```python
from build123d import *

# Parameters (mm, degrees)
BOSS_EXTRUDE1_DEPTH = 6.35
SKETCH2_W           = 17.78
SKETCH2_H           = 8.89
CUT_EXTRUDE1_DEPTH  = 6.35
SKETCH3_W           = 6.35
SKETCH3_H           = 6.35
BOSS_EXTRUDE2_DEPTH = 12.7


with BuildPart() as part:
    # Sketch1 → Boss-Extrude1 (new body)
    with BuildSketch(Plane(origin=(0, 0, 0), x_dir=(1, 0, 0), z_dir=(0, 1, 0))):
        with BuildLine():
            Line((9.525, -3.175), (-9.525, -3.175))
            Line((-9.525, -3.175), (-9.525, 3.175))
            Line((-9.525, 3.175), (-19.05, 3.175))
            Line((-19.05, 3.175), (-19.05, 28.575))
            ThreePointArc((-19.05, 28.575), (-15.330256121, 37.555256121), (-6.35, 41.275))
            Line((-6.35, 41.275), (6.35, 41.275))
            ThreePointArc((6.35, 41.275), (15.330256121, 37.555256121), (19.05, 28.575))
            Line((19.05, 28.575), (19.05, 3.175))
            Line((19.05, 3.175), (9.525, 3.175))
            Line((9.525, 3.175), (9.525, -3.175))
        make_face()
    extrude(amount=BOSS_EXTRUDE1_DEPTH)

    # Sketch2 → Cut-Extrude1 (cut)
    with BuildSketch(Plane(origin=(0, 6.35, 0), x_dir=(1, 0, 0), z_dir=(0, 1, 0))):
        with Locations((0, 11.43)):
            Rectangle(SKETCH2_W, SKETCH2_H)
    extrude(amount=-CUT_EXTRUDE1_DEPTH, mode=Mode.SUBTRACT)

    # Sketch3 → Boss-Extrude2 (add)
    with BuildSketch(Plane.XY.offset(3.175)):
        with Locations((-6.35, 3.175)):
            Rectangle(SKETCH3_W, SKETCH3_H)
        with Locations((6.35, 3.175)):
            Rectangle(SKETCH3_W, SKETCH3_H)
    extrude(amount=BOSS_EXTRUDE2_DEPTH)


solid = part.part
```
CAD build for the part. Positions are in the model's coordinates, mm. A direction names the side the tool comes from. Give positions to 0.01 mm unless a question says otherwise; leave off trailing zeros. Loops run counter-clockwise (first coordinate to the right, second up) from the corner with the lowest first, then second, coordinate; pieces in that order, holes last. Notation, with made-up numbers: (82.25, 22) -> (141.25, 22) arc R23 ccw to (141.25, 37) -> close; hole circle Ø2 at (12.25, -20.75). An arc over 180 degrees is marked (long way). Use a Markdown table: item, result.
1. Mould opens along X. For faces 1 (the flat face through (19.05, 3, -16)), 2 (the flat face through (14, 3, -3.175)), 3 (the flat face through (0, 3, -6.985)) say: pulls with the +X half, pulls with the -X half, needs draft (parallel to the pull), parting line crosses it, or undercut.
Check result:
| item | result |
|---|---|
| face 1 | pulls with the +X half |
| face 2 | needs draft |
| face 3 | undercut |
2. Slice it at D-D (x = 10.5). List the corners of the cut face in (y, z) (3 decimals).
Check result:
| item | result |
|---|---|
| outline | (0, -40.578) -> (6.35, -40.578) -> (6.35, -3.175) -> (0, -3.175) -> close |
3. Wall check: L1, parallel to X at y = 0.75, z = -11.5; L2, parallel to Z at x = -4.5, y = 4.75 (3 decimals); L3, parallel to Z at x = 0, y = 2.5 (3 decimals). Give the ranges that are in metal, low to high. Write a range as [from, to].
Check result:
| item | result |
|---|---|
| L1 | x = [-19.05, -8.89], [8.89, 19.05] |
| L2 | z = [-41.275, -15.875], [-6.985, 15.875] |
| L3 | z = [-41.275, -15.875], [-6.985, 3.175] |
4. Slice it at C-C (x = -4.5). List the corners of the cut face in (y, z) (3 decimals).
Check result:
| item | result |
|---|---|
| outline | (0, -41.275) -> (6.35, -41.275) -> (6.35, -15.875) -> (0, -15.875) -> close; (0, -6.985) -> (6.35, -6.985) -> (6.35, 15.875) -> (0, 15.875) -> close |
5. Slice it at B-B (y = 5.5). List the corners of the cut face in (x, z) (3 decimals).
Check result:
| item | result |
|---|---|
| outline | (-19.05, -28.575) arc R12.7 ccw to (-6.35, -41.275) -> (6.35, -41.275) arc R12.7 ccw to (19.05, -28.575) -> (19.05, -3.175) -> (9.525, -3.175) -> (9.525, 15.875) -> (3.175, 15.875) -> (3.175, 3.175) -> (-3.175, 3.175) -> (-3.175, 15.875) -> (-9.525, 15.875) -> (-9.525, -3.175) -> (-19.05, -3.175) -> close; hole (-8.89, -15.875) -> (8.89, -15.875) -> (8.89, -6.985) -> (-8.89, -6.985) -> close |
6. Slice it at A-A (z = -12.5). List the corners of the cut face in (x, y), plus the area to 3 significant figures.
Check result:
| item | result |
|---|---|
| outline | (-19.05, 0) -> (-8.89, 0) -> (-8.89, 6.35) -> (-19.05, 6.35) -> close; (8.89, 0) -> (19.05, 0) -> (19.05, 6.35) -> (8.89, 6.35) -> close |
| area | 129 mm^2 |
7. Flat gauge pins, fed straight in: pin 1 (1.9 mm diameter, centred on y = 4.5, z = 7, fed in from -X) (3 decimals); pin 2 (1.9 mm diameter, centred on y = 3.5, z = 9.5, fed in from +X) (3 decimals); pin 3 (1.9 mm diameter, centred on x = -13, y = 4, fed in from +Z) (3 decimals). Where does each tip first touch, or does it go through?
Check result:
| item | result |
|---|---|
| pin 1 | stops at x = -9.525 |
| pin 2 | stops at x = 9.525 |
| pin 3 | stops at z = -3.175 |
8. Which spindle directions (+Z, -Z, +X, -X, +Y, -Y) get a long thin tool onto all of the face, cutting with end or side? Do faces 4 (the flat face through (-8.89, 3, -11)), 5 (the flat face through (0, 3, 3.175)), 6 (the flat face through (0, 0, -19)), 7 (the flat face through (0, 3, -41.275)), 8 (the flat face through (-14, 3, -3.175)). Say none if no direction does.
Check result:
| item | result |
|---|---|
| face 4 | +Y, -Y |
| face 5 | +Z, +Y, -Y |
| face 6 | +Z, -Z, +X, -X, -Y |
| face 7 | -Z, +X, -X, +Y, -Y |
| face 8 | +Z, -X, +Y, -Y |
